Geometry: final body of the model. Coordinates: model frame, mm. Round coordinates to 2 decimals unless told otherwise and drop trailing zeros. Write each loop counter-clockwise with the first axis right and the second up, starting at its lowest first coordinate (ties: lowest second). Pieces come first, ordered by that corner, then holes.
from build123d import *

# Parameters (mm, degrees)
CHAFL_N2_SIZE = 0.5


with BuildPart() as part:
    # Croquis1 → Revolución1 (revolve)
    with BuildSketch(Plane(origin=(0, -190, 0), x_dir=(1, 0, 0), z_dir=(0, 1, 0))):
        with BuildLine():
            Line((6.5, 0), (6.5, 0.75))
            ThreePointArc((6.5, 0.75), (5.25, 2), (6.5, 3.25))
            Line((6.5, 3.25), (6.5, 4))
            Line((6.5, 4), (1.995632004, 4))
            Line((1.995632004, 4), (1.995632004, 0))
            Line((1.995632004, 0), (6.5, 0))
        make_face()
    revolve(axis=Axis((0, -190, -5), (0, 0, 1)))

    # Chaflán2
    chafl_n2_edges = [part.edges().sort_by_distance(p)[0] for p in [
        (-1.995632004, -190, 0),
        (-1.995632004, -190, -4),
    ]]
    chamfer(chafl_n2_edges, length=CHAFL_N2_SIZE)


solid = part.part
1) Section B-B on y = -190. Output: boundary loops of the cut face in (x, z).
2) First-contact query: P1, Ø1.5, axis at x = 3.5, z = -3.5, coming from the -Y side; P2, Ø2, axis at x = -2, z = -2, coming from the +Y side. Flat tips, straight axial feed; report the tip coordinate or a pass-through.
3) Section A-A on x = 0. Output: boundary loops of the cut face in (y, z), plus the area to 3 significant figures.
4) Line query: probe 1 along Y at (x, z) = (0, -1.8); probe 2 along X at (y, z) = (-190.75, -0.6); probe 3 along Z at (x, y) = (5.5, -191.5). Output: solid intervals per line, ascending.
5) Section C-C on z = -1.55. Output: boundary loops of the cut face in (x, y).
6) Draft query along X for faces 1 (the cylindrical face through (-0.43, -191.95, -1.98)), 2 (the flat face through (0, -193, 0)), 3 (the cylindrical face through (-1.409, -196.345, -3.63)). Return one class per face: pulls with the +X half, pulls with the -X half, needs draft (parallel to the pull), parting line crosses it, or undercut.
Filled in:
1. outline: (-6.5, -4) - (-2.5, -4) - (-2, -3.5) - (-2, -0.5) - (-2.5, 0) - (-6.5, 0) - (-6.5, -0.75) arc R1.25 cw to (-6.5, -3.25) - close; (2, -3.5) - (2.5, -4) - (6.5, -4) - (6.5, -3.25) arc R1.25 cw to (6.5, -0.75) - (6.5, 0) - (2.5, 0) - (2, -0.5) - close
2. P1: stops at y = -195.89
2. P2: stops at y = -184.57
3. outline: (-196.5, -4) - (-192.5, -4) - (-192, -3.5) - (-192, -0.5) - (-192.5, 0) - (-196.5, 0) - (-196.5, -0.75) arc R1.25 cw to (-196.5, -3.25) - close; (-188, -3.5) - (-187.5, -4) - (-183.5, -4) - (-183.5, -3.25) arc R1.25 cw to (-183.5, -0.75) - (-183.5, 0) - (-187.5, 0) - (-188, -0.5) - close
3. area: 30.6 mm2
4. probe 1: y = -195.27 to -192, -188 to -184.73
4. probe 2: x = -6.46 to -1.85, 1.85 to 6.46
4. probe 3: z = -4 to -2.96, -1.04 to 0
5. outline: circle Ø10.67 at (0, -190); hole circle Ø3.99 at (0, -190)
6. face 1: undercut
6. face 2: needs draft
6. face 3: parting line crosses it
